Print and shaded views of the part. All mm, measured from the part's lowest x, y and z. Round coordinates to 2 decimals unless told otherwise and drop trailing zeros. Write each loop counter-clockwise with the first axis right and the second up, starting at its lowest first coordinate (ties: lowest second). Pieces come first, ordered by that corner, then holes. Notation, with made-up numbers: (3.5, -25) - (39.5, -25) arc R15 cw to (39.5, -19) - close; hole circle Ø8 at (64.5, 17). An arc over 180 degrees is marked (long way). One line per item, written item: value.
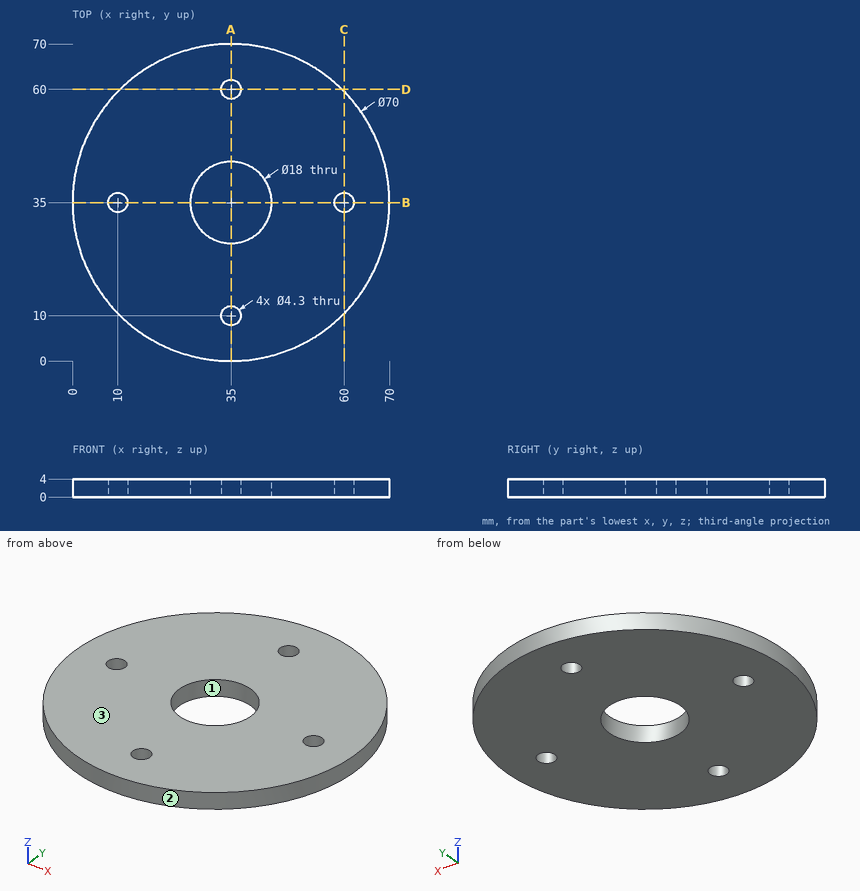
1. Band-saw the part on A-A on x = 35. Write the cut outline in (y, z).
Report:
outline: (0, 0) - (7.85, 0) - (7.85, 4) - (0, 4) - close; (12.15, 0) - (26, 0) - (26, 4) - (12.15, 4) - close; (44, 0) - (57.85, 0) - (57.85, 4) - (44, 4) - close; (62.15, 0) - (70, 0) - (70, 4) - (62.15, 4) - close
2. Drop flat-ended pins along their axis: pin 1 (2.5 mm diameter, centred on x = 35, y = 60, fed in from -Z); pin 2 (1.5 mm diameter, centred on y = 38.5, z = 0.5, fed in from +X); pin 3 (2 mm diameter, centred on x = 44, z = 2, fed in from -Y). Give the stop position or say it passes through.
Report:
pin 1: through
pin 2: x = 69.89
pin 3: y = 0.93
3. Band-saw the part on C-C on x = 60. Write the cut outline in (y, z), plus the area to 3 significant figures.
Report:
outline: (10.51, 0) - (32.85, 0) - (32.85, 4) - (10.51, 4) - close; (37.15, 0) - (59.49, 0) - (59.49, 4) - (37.15, 4) - close
area: 179 mm²
4. Mould opens along X. For the marked faces 1, 2 and 3 say: released by +X, released by -X, zero draft, split by the parting line, or undercut.
Report:
face 1: undercut
face 2: split by the parting line
face 3: zero draft
5. Wall check: probe 1 along Y at (x, z) = (35, 1.55); probe 2 along Y at (x, z) = (36.5, 1.35); probe 3 along Y at (x, z) = (10, 2.9). Give the ranges that are in metal, low to high. Write a range as [from, to].
Report:
probe 1: [0, 7.85], [12.15, 26], [44, 57.85], [62.15, 70]
probe 2: [0.03, 8.46], [11.54, 26.13], [43.87, 58.46], [61.54, 69.97]
probe 3: [10.51, 32.85], [37.15, 59.49]
